```python
from build123d import *

# Parameters (mm, degrees)
SKETCH1_W           = 40
SKETCH1_H           = 20
BOSS_EXTRUDE1_DEPTH = 3
SNAP_START          = -1.4
SNAP_HOOK1_DEPTH    = 2.95
SNAP_START_2        = -8.315183144
SNAP_HOOK1_2_DEPTH  = 16.630366288
SNAP_START_3        = -5.859491926
SNAP_HOOK1_3_DEPTH  = 11.718983852
SNAP_START_4        = -6
SNAP_HOOK1_4_DEPTH  = 14
FILLET1_R           = 1
CUT_EXTRUDE1_REACH  = 37.057
SKETCH3_R           = 1.5
FILLET2_R           = 1


with BuildPart() as part:
    # Sketch1 → Boss-Extrude1 (new body)
    with BuildSketch(Plane.XY):
        Rectangle(SKETCH1_W, SKETCH1_H)
    extrude(amount=BOSS_EXTRUDE1_DEPTH)

    # Snap Hook1: read off the stored shape, not the designer's step
    # Snap Hook1 outline → Snap Hook1 (add)
    with BuildSketch(Plane(origin=(0, 0, 0), x_dir=(1, 0, 0), z_dir=(0, 1, 0)).offset(SNAP_START)):
        Polygon((8.315183144, -3), (-8.315183144, -3), (-5, -30), (5, -30), align=None)
    extrude(amount=SNAP_HOOK1_DEPTH)

    # Snap Hook1 2 outline → Snap Hook1 2 (add)
    with BuildSketch(Plane.YZ.offset(SNAP_START_2)):
        Polygon((-1.4, 3), (-1.4, 30), (-5.45, 3), align=None)
    extrude(amount=SNAP_HOOK1_2_DEPTH)

    # Snap Hook1 3 outline → Snap Hook1 3 (add)
    with BuildSketch(Plane.YZ.offset(SNAP_START_3)):
        Polygon((1.55, 30), (1.55, 23), (6.55, 23), (6.55, 25), align=None)
    extrude(amount=SNAP_HOOK1_3_DEPTH)

    # Snap Hook1 4 outline → Snap Hook1 4 (cut)
    with BuildSketch(Plane(origin=(0, 0, 0), x_dir=(1, 0, 0), z_dir=(0, 1, 0)).offset(SNAP_START_4)):
        Polygon((-8.315183144, -3), (-8.315183144, -31), (-4.877215439, -31), (-5, -30), align=None)
        Polygon((5, -30), (4.877215439, -31), (8.315183144, -31), (8.315183144, -3), align=None)
    extrude(amount=SNAP_HOOK1_4_DEPTH, mode=Mode.SUBTRACT)

    # Fillet1
    # the kernel refuses this fillet: 1 mm, written as the material it adds along each edge
    with BuildSketch(Plane(origin=(10.815183144, 1.55, 3), x_dir=(0, 1, 0), z_dir=(-1, 0, 0))) as fillet1_piece_1_section:
        with BuildLine():
            CenterArc((FILLET1_R, -FILLET1_R), FILLET1_R, 90, 90)
            Line((0, -FILLET1_R), (0, 0))
            Line((0, 0), (FILLET1_R, 0))
        make_face()
    fillet1_piece_1 = extrude(amount=21.630366288, mode=Mode.PRIVATE)
    fillet1_piece_1 = split(fillet1_piece_1, bisect_by=Plane(origin=(-8.031056326, 1.55, 5.314027238), z_dir=(0.9925461516430047, 0, -0.12186934339144287)), keep=Keep.TOP, mode=Mode.PRIVATE)
    fillet1_piece_1 = split(fillet1_piece_1, bisect_by=Plane(origin=(8.352313486, 1.55, 2.697597631), z_dir=(-0.9925461516430047, 0, -0.12186934339144287)), keep=Keep.TOP, mode=Mode.PRIVATE)
    add(fillet1_piece_1)
    with BuildSketch(Plane(origin=(8.315183144, 1.55, 3), x_dir=(1, 0, 0), z_dir=(0, -1, 0))) as fillet1_piece_2_section:
        with BuildLine():
            CenterArc((FILLET1_R * 0.884725264568, FILLET1_R), FILLET1_R, 186.999999999, 83.000000001)
            Line((-FILLET1_R * 0.107820887075, FILLET1_R * 0.878130656609), (0, 0))
            Line((0, 0), (FILLET1_R * 0.884725264568, 0))
        make_face()
    fillet1_piece_2 = extrude(amount=9.211813161, mode=Mode.PRIVATE)
    fillet1_piece_2 = split(fillet1_piece_2, bisect_by=Plane(origin=(8.315183144, -5.29596577, 4.026894866), z_dir=(0, 0.9889363528682975, -0.14834045293024464)), keep=Keep.TOP, mode=Mode.PRIVATE)
    add(fillet1_piece_2)
    with BuildSketch(Plane(origin=(-10.468151696, -5.45, 3), x_dir=(0, -1, 0), z_dir=(1, 0, 0))) as fillet1_piece_3_section:
        with BuildLine():
            CenterArc((FILLET1_R * 0.861187420808, -FILLET1_R), FILLET1_R, 90, 81.46923439)
            Line((-FILLET1_R * 0.12774893206, -FILLET1_R * 0.85165954707), (0, 0))
            Line((0, 0), (FILLET1_R * 0.861187420808, 0))
        make_face()
    fillet1_piece_3 = extrude(amount=20.936303392, mode=Mode.PRIVATE)
    fillet1_piece_3 = split(fillet1_piece_3, bisect_by=Plane(origin=(-8.347159328, -5.45, 2.739574883), z_dir=(0.9925461516430047, 0, -0.12186934339144287)), keep=Keep.TOP, mode=Mode.PRIVATE)
    fillet1_piece_3 = split(fillet1_piece_3, bisect_by=Plane(origin=(8.036210484, -5.45, 5.272049985), z_dir=(-0.9925461516430047, 0, -0.12186934339144287)), keep=Keep.TOP, mode=Mode.PRIVATE)
    add(fillet1_piece_3)
    with BuildSketch(Plane(origin=(-8.315183144, -7.661813161, 3), x_dir=(-1, 0, 0), z_dir=(0, 1, 0))) as fillet1_piece_4_section:
        with BuildLine():
            CenterArc((FILLET1_R * 0.884725264568, FILLET1_R), FILLET1_R, 186.999999999, 83.000000001)
            Line((-FILLET1_R * 0.107820887075, FILLET1_R * 0.878130656609), (0, 0))
            Line((0, 0), (FILLET1_R * 0.884725264568, 0))
        make_face()
    fillet1_piece_4 = extrude(amount=9.211813161, mode=Mode.PRIVATE)
    fillet1_piece_4 = split(fillet1_piece_4, bisect_by=Plane(origin=(-8.315183144, -5.498670705, 2.675528632), z_dir=(0, 0.9889363528682975, -0.14834045293024464)), keep=Keep.TOP, mode=Mode.PRIVATE)
    add(fillet1_piece_4)
    with BuildSketch(Plane(origin=(8.315183144, 3.761813161, 3), x_dir=(1, 0, 0), z_dir=(0, -1, 0))) as fillet1_piece_5a_section:
        with BuildLine():
            CenterArc((FILLET1_R * 0.884725264568, FILLET1_R), FILLET1_R, 186.999999999, 83.000000001)
            Line((-FILLET1_R * 0.107820887075, FILLET1_R * 0.878130656609), (0, 0))
            Line((0, 0), (FILLET1_R * 0.884725264568, 0))
        make_face()
    fillet1_piece_5a = extrude(amount=11.423626323, mode=Mode.PRIVATE)
    fillet1_piece_5a = split(fillet1_piece_5a, bisect_by=Plane(origin=(8.315183144, 1.55, 3), z_dir=(0, 1, 0)), keep=Keep.TOP, mode=Mode.PRIVATE)
    with BuildSketch(Plane(origin=(10.815183144, 1.55, 3), x_dir=(0, 1, 0), z_dir=(-1, 0, 0))) as fillet1_piece_5b_section:
        with BuildLine():
            CenterArc((FILLET1_R, -FILLET1_R), FILLET1_R, 90, 90)
            Line((0, -FILLET1_R), (0, 0))
            Line((0, 0), (FILLET1_R, 0))
        make_face()
    fillet1_piece_5b = extrude(amount=21.630366288, mode=Mode.PRIVATE)
    fillet1_piece_5b = split(fillet1_piece_5b, bisect_by=Plane(origin=(8.352313486, 1.55, 2.697597631), z_dir=(0.9925461516430047, 0, 0.12186934339144287)), keep=Keep.TOP, mode=Mode.PRIVATE)
    fillet1_piece_5 = fillet1_piece_5a & fillet1_piece_5b
    add(fillet1_piece_5)
    with BuildSketch(Plane(origin=(10.815183144, 1.55, 3), x_dir=(0, 1, 0), z_dir=(-1, 0, 0))) as fillet1_piece_6a_section:
        with BuildLine():
            CenterArc((FILLET1_R, -FILLET1_R), FILLET1_R, 90, 90)
            Line((0, -FILLET1_R), (0, 0))
            Line((0, 0), (FILLET1_R, 0))
        make_face()
    fillet1_piece_6a = extrude(amount=21.630366288, mode=Mode.PRIVATE)
    fillet1_piece_6a = split(fillet1_piece_6a, bisect_by=Plane(origin=(-8.031056326, 1.55, 5.314027238), z_dir=(-0.9925461516430047, 0, 0.12186934339144287)), keep=Keep.TOP, mode=Mode.PRIVATE)
    with BuildSketch(Plane(origin=(-8.315183144, -7.661813161, 3), x_dir=(-1, 0, 0), z_dir=(0, 1, 0))) as fillet1_piece_6b_section:
        with BuildLine():
            CenterArc((FILLET1_R * 0.884725264568, FILLET1_R), FILLET1_R, 186.999999999, 83.000000001)
            Line((-FILLET1_R * 0.107820887075, FILLET1_R * 0.878130656609), (0, 0))
            Line((0, 0), (FILLET1_R * 0.884725264568, 0))
        make_face()
    fillet1_piece_6b = extrude(amount=11.423626323, mode=Mode.PRIVATE)
    fillet1_piece_6b = split(fillet1_piece_6b, bisect_by=Plane(origin=(-8.315183144, 1.55, 3), z_dir=(0, 1, 0)), keep=Keep.TOP, mode=Mode.PRIVATE)
    fillet1_piece_6 = fillet1_piece_6a & fillet1_piece_6b
    add(fillet1_piece_6)
    with BuildSketch(Plane(origin=(-10.468151696, -5.45, 3), x_dir=(0, -1, 0), z_dir=(1, 0, 0))) as fillet1_piece_7a_section:
        with BuildLine():
            CenterArc((FILLET1_R * 0.861187420808, -FILLET1_R), FILLET1_R, 90, 81.46923439)
            Line((-FILLET1_R * 0.12774893206, -FILLET1_R * 0.85165954707), (0, 0))
            Line((0, 0), (FILLET1_R * 0.861187420808, 0))
        make_face()
    fillet1_piece_7a = extrude(amount=20.936303392, mode=Mode.PRIVATE)
    fillet1_piece_7a = split(fillet1_piece_7a, bisect_by=Plane(origin=(8.036210484, -5.45, 5.272049985), z_dir=(0.9925461516430047, 0, 0.12186934339144287)), keep=Keep.TOP, mode=Mode.PRIVATE)
    with BuildSketch(Plane(origin=(8.315183144, 1.55, 3), x_dir=(1, 0, 0), z_dir=(0, -1, 0))) as fillet1_piece_7b_section:
        with BuildLine():
            CenterArc((FILLET1_R * 0.884725264568, FILLET1_R), FILLET1_R, 186.999999999, 83.000000001)
            Line((-FILLET1_R * 0.107820887075, FILLET1_R * 0.878130656609), (0, 0))
            Line((0, 0), (FILLET1_R * 0.884725264568, 0))
        make_face()
    fillet1_piece_7b = extrude(amount=9.211813161, mode=Mode.PRIVATE)
    fillet1_piece_7b = split(fillet1_piece_7b, bisect_by=Plane(origin=(8.315183144, -5.29596577, 4.026894866), z_dir=(0, -0.9889363528682975, 0.14834045293024464)), keep=Keep.TOP, mode=Mode.PRIVATE)
    fillet1_piece_7 = fillet1_piece_7a & fillet1_piece_7b
    add(fillet1_piece_7)
    with BuildSketch(Plane(origin=(-10.468151696, -5.45, 3), x_dir=(0, -1, 0), z_dir=(1, 0, 0))) as fillet1_piece_8a_section:
        with BuildLine():
            CenterArc((FILLET1_R * 0.861187420808, -FILLET1_R), FILLET1_R, 90, 81.46923439)
            Line((-FILLET1_R * 0.12774893206, -FILLET1_R * 0.85165954707), (0, 0))
            Line((0, 0), (FILLET1_R * 0.861187420808, 0))
        make_face()
    fillet1_piece_8a = extrude(amount=20.936303392, mode=Mode.PRIVATE)
    fillet1_piece_8a = split(fillet1_piece_8a, bisect_by=Plane(origin=(-8.347159328, -5.45, 2.739574883), z_dir=(-0.9925461516430047, 0, 0.12186934339144287)), keep=Keep.TOP, mode=Mode.PRIVATE)
    with BuildSketch(Plane(origin=(-8.315183144, -7.661813161, 3), x_dir=(-1, 0, 0), z_dir=(0, 1, 0))) as fillet1_piece_8b_section:
        with BuildLine():
            CenterArc((FILLET1_R * 0.884725264568, FILLET1_R), FILLET1_R, 186.999999999, 83.000000001)
            Line((-FILLET1_R * 0.107820887075, FILLET1_R * 0.878130656609), (0, 0))
            Line((0, 0), (FILLET1_R * 0.884725264568, 0))
        make_face()
    fillet1_piece_8b = extrude(amount=9.211813161, mode=Mode.PRIVATE)
    fillet1_piece_8b = split(fillet1_piece_8b, bisect_by=Plane(origin=(-8.315183144, -5.498670705, 2.675528632), z_dir=(0, -0.9889363528682975, 0.14834045293024464)), keep=Keep.TOP, mode=Mode.PRIVATE)
    fillet1_piece_8 = fillet1_piece_8a & fillet1_piece_8b
    add(fillet1_piece_8)

    # Sketch3 → Cut-Extrude1 (cut, up to next)
    with BuildSketch(Plane.XY.offset(3), mode=Mode.PRIVATE) as cut_extrude1_sk1:
        with Locations((-14.599954204, 0)):
            Circle(SKETCH3_R)
    cut_extrude1_tool1 = extrude(cut_extrude1_sk1.sketch, amount=-CUT_EXTRUDE1_REACH, mode=Mode.PRIVATE) & part.part
    cut_extrude1 = cut_extrude1_tool1.solids().sort_by_distance((-14.599954, 0, 3))[0]
    add(cut_extrude1, mode=Mode.SUBTRACT)

    # Mirror1: Cut-Extrude1 across plane
    add(cut_extrude1.mirror(Plane(origin=(0, 0, 0), x_dir=(0, 0, 1), z_dir=(1, 0, 0))), mode=Mode.SUBTRACT)

    # Fillet2
    fillet2_edges = [part.edges().sort_by_distance(p)[0] for p in [
        (20, -10, 1.5),
        (-20, -10, 1.5),
        (-20, 10, 1.5),
        (20, 10, 1.5),
    ]]
    fillet(fillet2_edges, radius=FILLET2_R)


solid = part.part
```
Work out the finished part from the listing and answer in its coordinate system (mm). A direction names the side the tool comes from. Give positions to 0.01 mm unless a question says otherwise; leave off trailing zeros. Order: outer loops, then holes, each group sorted by start corner. A loop starts at its lowest first (then second) coordinate and runs counter-clockwise, first axis right, second up. Notation, with made-up numbers: M 83,12.25 L 135,12.25 A29 cw 135,35.25 Z; hole C 57.25,85 d10. An arc over 180 degrees is marked long. Return JSON: item names as keys, results as strings.
1) Section C-C, the plane x = 2 is taken. Write down the section's boundary in (y, z).
Resolved:
{"outline": "M -10,0 L 10,0 L 10,3 L 2.55,3 A1 cw 1.55,4 L 1.55,23 L 6.55,23 L 6.55,25 L 1.55,30 L -1.4,30 L -5.32,3.85 A1 cw -6.31,3 L -10,3 Z"}
2) Straight lines are drawn through the part: line 1 along Z through (x, y) = (11, -6); line 2 along Z through (x, y) = (-2.5, 6); line 3 along Z through (x, y) = (1.5, 4.5). For each, find the intervals that lie inside material, in ascending order. Write a range as [from, to].
Resolved:
{"line 1": "[0, 3]", "line 2": "[0, 3], [23, 25.55]", "line 3": "[0, 3], [23, 27.05]"}
3) Each of these flat-tipped pins is pushed along its axis until it touches: pin 1 (3 mm diameter, centred on y = 3, z = 13, fed in from +X); pin 2 (4 mm diameter, centred on x = -9.5, z = 8, fed in from -Y); pin 3 (5 mm diameter, centred on y = 3, z = 16.5, fed in from +X). Where does it stop, or does it pass through?
Resolved:
{"pin 1": "x = 7.13", "pin 2": "y = -4.87", "pin 3": "x = 6.91"}
4) Section B-B, the plane y = 3.75 is taken. Write down the section's boundary in (x, z).
Resolved:
{"outline": "M -20,0 L 20,0 L 20,3 L -20,3 Z; M -5.86,23 L 5.86,23 L 5.27,27.8 L -5.27,27.8 Z"}
5) A tool of negligible diameter and unlimited length cuts with its end or side. For faces 1 (the cylindrical face through (0.129, 1.851, 3.285)), 2 (the flat face through (0, 6.55, 24)), 3 (the cylindrical face through (19.699, -9.715, 1.521)), from which of +Z, -Z, +X, -X, +Y, -Y can it reach the whole face along a straight path? Write none if from no direction.
Resolved:
{"face 1": "+X, -X, +Y", "face 2": "+Z, +X, -X, +Y", "face 3": "+Z, -Z, +X, -Y"}
6) For a pull along Y with two mould halves and no side action, classify faces 4 (the cylindrical face through (16.1, 0.07, 1.52)), 5 (the flat face through (0, 10, 1)), 6 (the flat face through (6.58, -0.79, 17.12)) as +Y half, -Y half, draft (parallel to the pull), parting line (faces both ways), or undercut.
Resolved:
{"face 4": "undercut", "face 5": "+Y half", "face 6": "draft"}
7) Section A-A, the plane y = 0 is taken. Write down the section's boundary in (x, z), plus the area to 3 significant figures.
Resolved:
{"outline": "M -20,0 L -16.1,0 L -16.1,3 L -20,3 Z; M -13.1,0 L 13.1,0 L 13.1,3 L 9.2,3 A1 cw 8.21,3.88 L 5,30 L -5,30 L -8.21,3.88 A1 cw -9.2,3 L -13.1,3 Z; M 16.1,0 L 20,0 L 20,3 L 16.1,3 Z", "area": "462 mm^2"}
8) Section D-D, the plane y = -4.5 is taken. Write down the section's boundary in (x, z).
Resolved:
{"outline": "M -20,0 L 20,0 L 20,3 L 9.2,3 A1 cw 8.21,3.88 L 7.54,9.33 L -7.54,9.33 L -8.21,3.88 A1 cw -9.2,3 L -20,3 Z"}
